Here's the drawing with two shaded views (mm, measured from the low corner). I have some questions. Coordinates: 2 decimals unless noted, no trailing zeros. Loops run counter-clockwise (first coordinate to the right, second up) from the corner with the lowest first, then second, coordinate; pieces in that order, holes last.
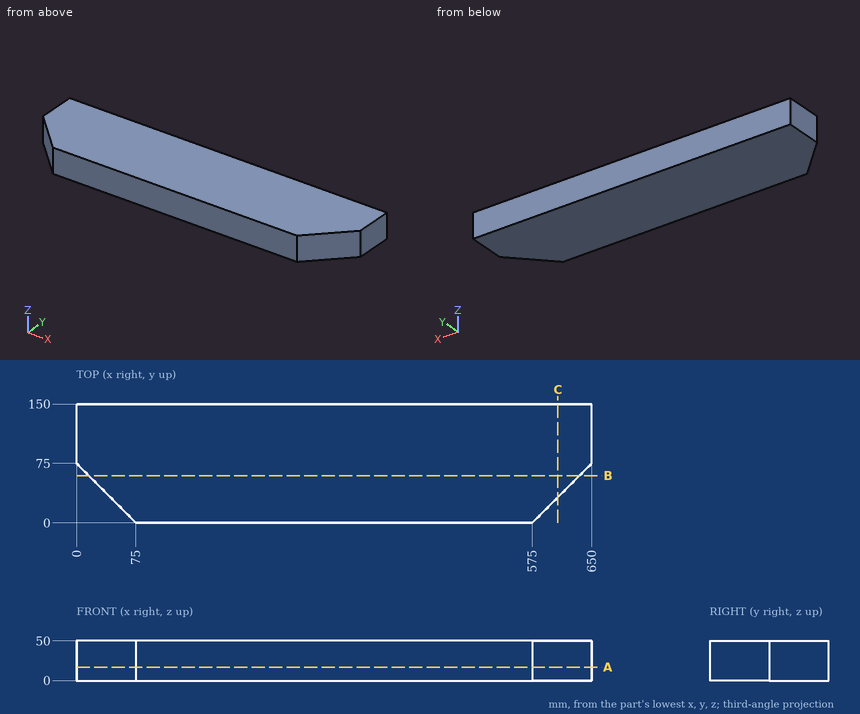
(1) I'm going to push flat-ended pins straight in: pin 1 (5 mm diameter, centred on y = 57, z = 42, fed in from -X); pin 2 (2 mm diameter, centred on y = 47, z = 20.5, fed in from -X); pin 3 (1.5 mm diameter, centred on y = 33.5, z = 20, fed in from +X). Where does each tip first touch, or does it pass through?
Check values:
pin 1: stops at x = 15.5
pin 2: stops at x = 27
pin 3: stops at x = 609.25
(2) If I drill on probe 1 along Y at (x, z) = (33, 30); probe 2 along X at (y, z) = (26.5, 30.5); probe 3 along X at (y, z) = (48, 38), over which ranges is the centre line in solid material (lowest first)?
Check values:
probe 1: y = 42 to 150
probe 2: x = 48.5 to 601.5
probe 3: x = 27 to 623
(3) I want a section at A-A on z = 17. Write out the boundary of the cut face in (x, y).
Check values:
outline: (0, 75) - (75, 0) - (575, 0) - (650, 75) - (650, 150) - (0, 150) - close
(4) I want a section at C-C on x = 607.5. Write out the boundary of the cut face in (y, z), then the cut area to 4 significant figures.
Check values:
outline: (32.5, 0) - (150, 0) - (150, 50) - (32.5, 50) - close
area: 5,875 mm2
(5) I want a section at B-B on y = 59.5. Write out the boundary of the cut face in (x, z).
Check values:
outline: (15.5, 0) - (634.5, 0) - (634.5, 50) - (15.5, 50) - close
